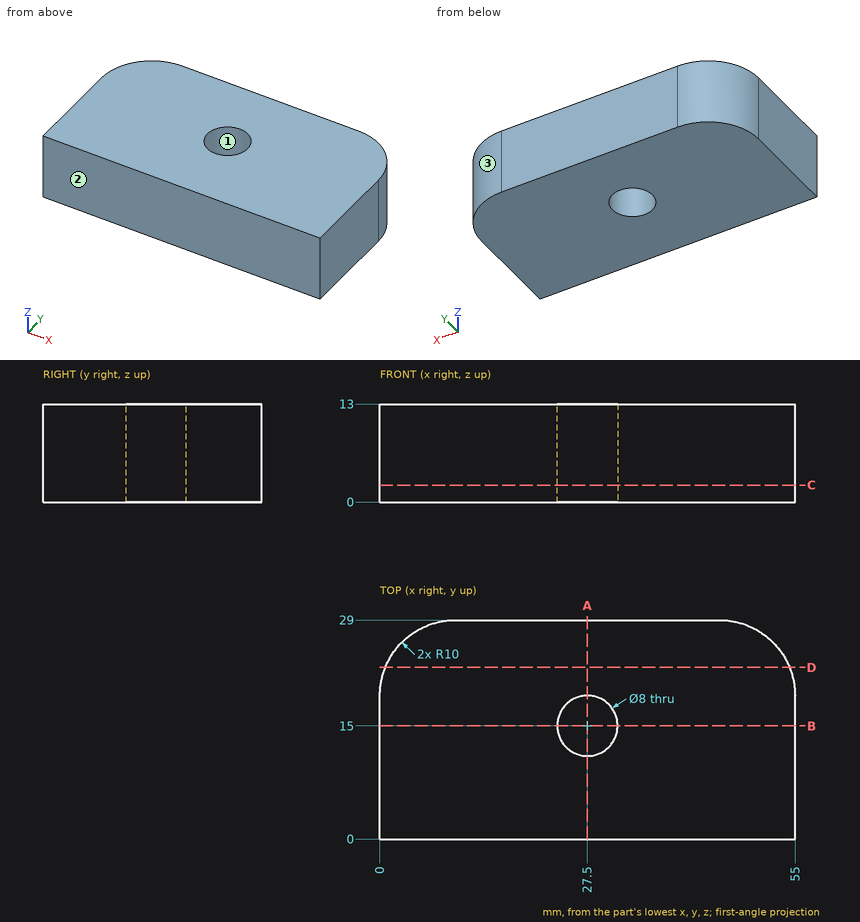
Source: three-view drawing plus pictorial views. Frame: mm from the lowest corner of the part. Coordinates: 2 decimals unless noted, no trailing zeros. Loops run counter-clockwise (first coordinate to the right, second up) from the corner with the lowest first, then second, coordinate; pieces in that order, holes last. Notation, with made-up numbers: (-25, 17) - (-17, 17) arc R20 cw to (-17, 51) - close; hole circle Ø2 at (10.25, 17.5). An arc over 180 degrees is marked (long way). Answer in a Markdown table with one row per item. Add a question column.
Item 1: Section query D-D on y = 22.75. Return the cut outline in (x, z), then the cut area to 3 significant figures.
Item 2: Contact query for a flat-ended pin moving along its axis: P1, Ø5, axis at x = 49.5, z = 2, coming from the +Y side. Output: stop coordinate, or through.
Item 3: Section query B-B on y = 15. Return the cut outline in (x, z), then the cut area to 3 significant figures.
Item 4: Mould query, pull axis X, two halves, no side actions, for the marked faces 1, 2 and 3. Classes: released by +X, released by -X, zero draft, split by the parting line, or undercut.
Item 5: Section query A-A on x = 27.5. Return the cut outline in (y, z), then the cut area to 3 significant figures.
Item 6: Line query: line 1 along Y through (x, z) = (27.5, 3.5); line 2 along X through (y, z) = (18.5, 7.25); line 3 along Y through (x, z) = (30, 1.75). Output: solid intervals per line, ascending. Write a range as [from, to].
Item 7: Section query C-C on z = 2.25. Return the cut outline in (x, y), then the cut area to 3 significant figures.
Recorded:
| question | item | result |
|---|---|---|
| 1 | outline | (0.73, 0) - (54.27, 0) - (54.27, 13) - (0.73, 13) - close |
| 1 | area | 696 mm^2 |
| 2 | P1 | y = 28.8 |
| 3 | outline | (0, 0) - (23.5, 0) - (23.5, 13) - (0, 13) - close; (31.5, 0) - (55, 0) - (55, 13) - (31.5, 13) - close |
| 3 | area | 611 mm^2 |
| 4 | face 1 | undercut |
| 4 | face 2 | zero draft |
| 4 | face 3 | released by +X |
| 5 | outline | (0, 0) - (11, 0) - (11, 13) - (0, 13) - close; (19, 0) - (29, 0) - (29, 13) - (19, 13) - close |
| 5 | area | 273 mm^2 |
| 6 | line 1 | [0, 11], [19, 29] |
| 6 | line 2 | [0, 25.56], [29.44, 55] |
| 6 | line 3 | [0, 11.88], [18.12, 29] |
| 7 | outline | (0, 0) - (55, 0) - (55, 19) arc R10 ccw to (45, 29) - (10, 29) arc R10 ccw to (0, 19) - close; hole circle Ø8 at (27.5, 15) |
| 7 | area | 1,500 mm^2 |
